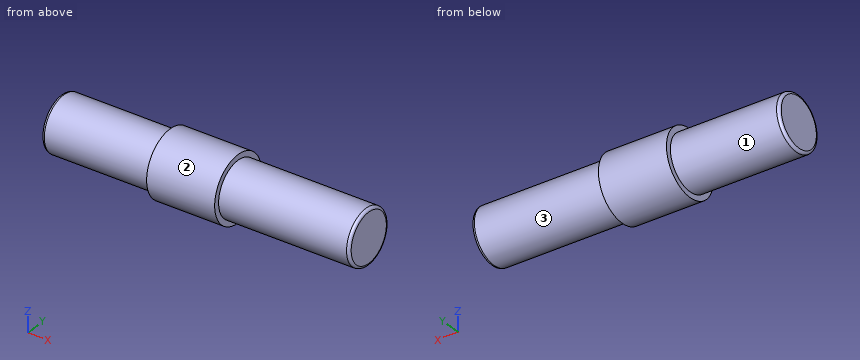
```python
from build123d import *

# Parameters (mm, degrees)
VERRUNDUNG1_R = 0.5


with BuildPart() as part:
    # Skizze1 → Rotation1 (revolve)
    with BuildSketch(Plane.XY):
        Polygon((-57.468382115, 0), (-57.468382115, 5), (-37.468382115, 5), (-37.468382115, 6), (-24.968382115, 6), (-24.968382115, 5), (-0.968382115, 5), (-0.968382115, 0), align=None)
    revolve(axis=Axis((-0.968382115, 0, 0), (-1, 0, 0)))

    # Verrundung1
    verrundung1_edges = [part.edges().sort_by_distance(p)[0] for p in [
        (-0.968382115, -5, 0),
        (-57.468382115, -5, 0),
    ]]
    fillet(verrundung1_edges, radius=VERRUNDUNG1_R)


solid = part.part
```
For this review, take the finished solid that the model builds, in its own axes (mm). Face numbers are marked on the shaded views. A direction names the side the tool comes from. Round coordinates to 2 decimals unless told otherwise and drop trailing zeros. Write each loop counter-clockwise with the first axis right and the second up, starting at its lowest first coordinate (ties: lowest second). Pieces come first, ordered by that corner, then holes. Notation, with made-up numbers: (55.5, -25) -> (95.5, -25) arc R27 ccw to (95.5, -3) -> close; hole circle Ø11 at (-10.5, 27.25). An arc over 180 degrees is marked (long way). Use one line per item in the form item = value.
Q1. Clearance check with flat-ended pins moving along their axes: pin 1 Ø1.5 at (x, z) = (-14, 4) entering from +Y; pin 2 Ø1.5 at (x, z) = (-17, -1) entering from +Y; pin 3 Ø5 at (x, z) = (-24.5, 2.5) entering from +Y; pin 4 Ø5 at (x, z) = (-41.5, 4) entering from -Y. State where each tip first meets the part, or that it passes through.
Resolved:
pin_1 = 3.8
pin_2 = 4.99
pin_3 = 6
pin_4 = -4.77
Q2. Consider section D-D (x = -45.5). State the section outline as (y, z) points.
Resolved:
outline = circle Ø10 at (0, 0)
Q3. Consider section A-A (y = 0). State the section outline as (x, z) points.
Resolved:
outline = (-57.47, -4.5) arc R0.5 ccw to (-56.97, -5) -> (-37.47, -5) -> (-37.47, -6) -> (-24.97, -6) -> (-24.97, -5) -> (-1.47, -5) arc R0.5 ccw to (-0.97, -4.5) -> (-0.97, 4.5) arc R0.5 ccw to (-1.47, 5) -> (-24.97, 5) -> (-24.97, 6) -> (-37.47, 6) -> (-37.47, 5) -> (-56.97, 5) arc R0.5 ccw to (-57.47, 4.5) -> close
Q4. To check wall thickness, follow probe 1 along X at (y, z) = (5.25, -1.25); probe 2 along Z at (x, y) = (-53, 0.25); probe 3 along Y at (x, z) = (-21, 0). State the ranges of each line that lie inside material, in increasing order. Write a range as from..to.
Resolved:
probe_1 = -37.47..-24.97
probe_2 = -4.99..4.99
probe_3 = -5..5
Q5. Consider section C-C (x = -30). State the section outline as (y, z) points.
Resolved:
outline = circle Ø12 at (0, 0)
Q6. Machinability: for the marked faces 1, 2 and 3, which of the approach directions +Z, -Z, +X, -X, +Y, -Y give a long, thin tool a straight path to every point of the face, cutting with its end or side? Answer none if there is none.
Resolved:
face_1 = -X
face_2 = +X, -X
face_3 = +X
